Part model, mm, in its own coordinate system. Round coordinates to 2 decimals unless told otherwise and drop trailing zeros. Loops run counter-clockwise (first coordinate to the right, second up) from the corner with the lowest first, then second, coordinate; pieces in that order, holes last.
(1) Mould opens along Y. For faces 1 (the face through (-15, -74, 10)), 2 (the face through (-82.881, -1.915, 5.07)), 3 (the face through (95.38, 30.04, 4.93)) say: +Y half, -Y half, draft (parallel to the pull), parting line (faces both ways), or undercut.
(2) Cut at A-A on y = 0. List the corners of the cut face in (x, z), then the cut area to 3 significant figures.
(3) Cut at D-D on y = 87.5. List the corners of the cut face in (x, z).
(4) Cut at C-C on z = 7.5. Count the separate pieces of the cut face and the enclosed holes in it, then the cut area to 3 significant figures.
(5) Probe probe 1 along Y at (x, z) = (57.5, 1.5); probe 2 along Y at (x, z) = (12.5, 2.25); probe 3 along Y at (x, z) = (34, 5.25). List the from-to ranges inside material, lowest first.
(6) Flat gauge pins, fed straight in: pin 1 (4 mm diameter, centred on y = 15.5, z = 3.5, fed in from +X); pin 2 (1.5 mm diameter, centred on x = 72, z = 7.5, fed in from +Y); pin 3 (6 mm diameter, centred on y = 50.5, z = 9, fed in from -X). Where does each tip first touch, or does it go through?
from build123d import *

# Parameters (mm, degrees)
F0_R            = 100
F1_DEPTH        = 10
F2_R            = 75
F3_DEPTH        = 10.001
F4_R            = 5
F5_DEPTH        = 10.001
F5_COPIES_COUNT = 7
F5_COPIES_ANGLE = 270
F8_R            = 7.5
F9_DEPTH        = 10.001


# Not quite as in the source:
# - a pattern or mirror of a feature is missing from the dataset's text; its kind, count and spacing are read off the source's solid


with BuildPart() as f1:
    # F0 (on Top) → F1 (new body)
    with BuildSketch(Plane.XY):
        Circle(F0_R)
    extrude(amount=F1_DEPTH)

    # F2 (on face) → F3 (cut, through all)
    with BuildSketch(Plane.XY.offset(10)):
        Circle(F2_R)
    extrude(amount=-F3_DEPTH, mode=Mode.SUBTRACT)

    # F4 (on face) → F5 (cut, through all)
    with BuildSketch(Plane.XY.offset(10)):
        with Locations((-87.5, 0)):
            Circle(F4_R)
    f5 = extrude(amount=-F5_DEPTH, mode=Mode.SUBTRACT)

    # F5_copies: F5 ×7 about axis
    f5_copies_axis = Axis((0, 0, 0), (0, 0, 1))
    for i in range(1, F5_COPIES_COUNT):
        add(f5.rotate(f5_copies_axis, i * F5_COPIES_ANGLE / (F5_COPIES_COUNT - 1)), mode=Mode.SUBTRACT)

    # F8 (on face) → F9 (cut, through all)
    with BuildSketch(Plane.XY.offset(10)):
        with Locations((-61.8718433538, 61.8718433538)):
            Circle(F8_R)
    extrude(amount=-F9_DEPTH, mode=Mode.SUBTRACT)


solid = f1.part
Final values:
1. face 1: draft
1. face 2: undercut
1. face 3: parting line
2. outline: (-100, 0) - (-92.5, 0) - (-92.5, 10) - (-100, 10) - close; (-82.5, 0) - (-75, 0) - (-75, 10) - (-82.5, 10) - close; (75, 0) - (82.5, 0) - (82.5, 10) - (75, 10) - close; (92.5, 0) - (100, 0) - (100, 10) - (92.5, 10) - close
2. area: 300 mm2
3. outline: (-48.41, 0) - (-5, 0) - (-5, 10) - (-48.41, 10) - close; (5, 0) - (48.41, 0) - (48.41, 10) - (5, 10) - close
4. separate pieces: 1
4. enclosed holes: 9
4. area: 13,000 mm2
5. probe 1: y = -81.82 to -64.3, -59.45 to -48.15, 48.15 to 59.45, 64.3 to 81.82
5. probe 2: y = -99.22 to -73.95, 73.95 to 99.22
5. probe 3: y = -94.04 to -66.85, 66.85 to 94.04
6. pin 1: stops at x = 99.08
6. pin 2: stops at y = 70.17
6. pin 3: stops at x = -88
